from build123d import *

# Parameters (mm, degrees)
SKETCH_W      = 40
SKETCH_H      = 40
PAD_DEPTH     = 8
SKETCH002_R   = 12.6
HOLE001_DEPTH = 20.001
FILLET_R      = 2
SKETCH003_R   = 2.1
PAD001_DEPTH  = 2.1
SKETCH001_R   = 1.1
HOLE_DEPTH    = 10.101
SKETCH004_R   = 3.2
PAD002_DEPTH  = 15


with BuildPart() as part:
    # Sketch → Pad (new body)
    with BuildSketch(Plane.XY):
        Rectangle(SKETCH_W, SKETCH_H)
    extrude(amount=PAD_DEPTH)

    # Sketch002 → Hole001 (cut, through all)
    with BuildSketch(Plane.XY.offset(20)):
        Circle(SKETCH002_R)
    extrude(amount=-HOLE001_DEPTH, mode=Mode.SUBTRACT)

    # Fillet
    fillet_edges = [part.edges().sort_by_distance(p)[0] for p in [
        (20, 20, 4),
        (20, -20, 4),
        (-20, -20, 4),
        (-20, 20, 4),
    ]]
    fillet(fillet_edges, radius=FILLET_R)

    # Sketch003 (on Face2 of Fillet) → Pad001 (join)
    with BuildSketch(Plane(origin=(0, 0, 0), x_dir=(1, 0, 0), z_dir=(0, 0, -1))):
        with Locations((-12.25, 12.25)):
            Circle(SKETCH003_R)
        with Locations((12.25, 12.25)):
            Circle(SKETCH003_R)
        with Locations((-12.25, -12.25)):
            Circle(SKETCH003_R)
        with Locations((12.25, -12.25)):
            Circle(SKETCH003_R)
    extrude(amount=PAD001_DEPTH)

    # Sketch001 (on Face6 of Pad) → Hole (cut, through all)
    with BuildSketch(Plane.XY.offset(8)):
        with Locations((12.25, -12.25)):
            Circle(SKETCH001_R)
        with Locations((-12.25, -12.25)):
            Circle(SKETCH001_R)
        with Locations((-12.25, 12.25)):
            Circle(SKETCH001_R)
        with Locations((12.25, 12.25)):
            Circle(SKETCH001_R)
    extrude(amount=-HOLE_DEPTH, mode=Mode.SUBTRACT)

    # Sketch004 (on Face7 of Hole) → Pad002 (join)
    with BuildSketch(Plane.XZ.offset(20)):
        with Locations((0, 4.8)):
            Circle(SKETCH004_R)
    extrude(amount=PAD002_DEPTH)


solid = part.part
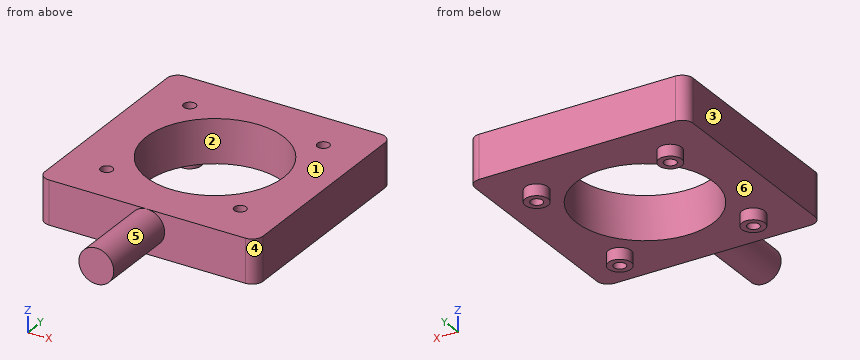
Here's how the part is built. I have some questions about the finished solid (model axes, mm). Face numbers are marked on the shaded views. A direction names the side the tool comes from. Round coordinates to 2 decimals unless told otherwise and drop trailing zeros. Write each loop counter-clockwise with the first axis right and the second up, starting at its lowest first coordinate (ties: lowest second). Pieces come first, ordered by that corner, then holes.
1. Suppose I cut it at B-B (z = 4.8). List the corners of the cut face in (x, y) for me, and give its area (3 significant figures).
2. Suppose I cut it at C-C (y = 1.5). List the corners of the cut face in (x, z) for me.
3. If we mould it in two halves opening along X, with no side actions, what happens to the marked faces 1, 2 and 3? For each: released by +X, released by -X, zero draft, split by the parting line, or undercut.
4. Will this pin go through, and if not, where does the flat tip stop? pin 1 Ø5 at (x, z) = (8, -1) entering from -Y.
5. Suppose I cut it at D-D (y = -17). List the corners of the cut face in (x, z) for me, and give its area (3 significant figures).
6. I need wall thicknesses on L1, parallel to Y at x = 0, z = 5; L2, parallel to X at y = 13, z = -1.5; L3, parallel to Z at x = 16, y = 3.5. Which ranges of each line are inside material? Lowest first, please.
7. Suppose I cut it at A-A (x = 9). List the corners of the cut face in (y, z) for me.
8. For the marked faces 4, 5 and 6, which set-ups out of +Z, -Z, +X, -X, +Y, -Y let a thin tool reach every point of the face, with its end or its side?
Answer sheet:
1. outline: (-20, -18) arc R2 ccw to (-18, -20) - (-3.2, -20) - (-3.2, -35) - (3.2, -35) - (3.2, -20) - (18, -20) arc R2 ccw to (20, -18) - (20, 18) arc R2 ccw to (18, 20) - (-18, 20) arc R2 ccw to (-20, 18) - close; hole circle Ø2.2 at (-12.25, -12.25); hole circle Ø2.2 at (-12.25, 12.25); hole circle Ø25.2 at (0, 0); hole circle Ø2.2 at (12.25, -12.25); hole circle Ø2.2 at (12.25, 12.25)
1. area: 1,180 mm2
2. outline: (-20, 0) - (-12.51, 0) - (-12.51, 8) - (-20, 8) - close; (12.51, 0) - (20, 0) - (20, 8) - (12.51, 8) - close
3. face 1: zero draft
3. face 2: undercut
3. face 3: released by -X
4. pin 1: stops at y = -20
5. outline: (-20, 0) - (20, 0) - (20, 8) - (-20, 8) - close
5. area: 320 mm2
6. L1: y = -35 to -12.6, 12.6 to 20
6. L2: x = -14.21 to -13.05, -11.45 to -10.29, 10.29 to 11.45, 13.05 to 14.21
6. L3: z = 0 to 8
7. outline: (-20, 0) - (-8.82, 0) - (-8.82, 8) - (-20, 8) - close; (8.82, 0) - (20, 0) - (20, 8) - (8.82, 8) - close
8. face 4: +Z, -Z, +X, -Y
8. face 5: -Y
8. face 6: -Z
